from build123d import *

# Parameters (mm, degrees)
SKETCH_W      = 98.2
SKETCH_H      = 92.2
SKETCH_R      = 5
SKETCH_R_2    = 3.2
SKETCH_R_3    = 1.4
SKETCH_R_4    = 2.2
SKETCH_W_2    = 79
SKETCH_H_2    = 52
PAD_DEPTH     = 1.8
SKETCH001_W   = 98.2
SKETCH001_H   = 92.2
SKETCH001_W_2 = 95
SKETCH001_H_2 = 89
PAD001_DEPTH  = 15.7
SKETCH002_R   = 4
SKETCH002_R_2 = 1.55
PAD002_DEPTH  = 6.2
FILLET_R      = 1.79
SKETCH003_W   = 27
SKETCH003_H   = 4
POCKET_DEPTH  = 1.6


with BuildPart() as part:
    # Sketch → Pad (new body)
    with BuildSketch(Plane.XY):
        Rectangle(SKETCH_W, SKETCH_H)
        with Locations((-37, -35)):
            Circle(SKETCH_R, mode=Mode.SUBTRACT)
        with Locations((-4, -35)):
            Circle(SKETCH_R_2, mode=Mode.SUBTRACT)
        with Locations((-23.1, -35)):
            Circle(SKETCH_R_3, mode=Mode.SUBTRACT)
        with Locations((-18.5, -30.4)):
            Circle(SKETCH_R_3, mode=Mode.SUBTRACT)
        with Locations((-13.9, -35)):
            Circle(SKETCH_R_3, mode=Mode.SUBTRACT)
        with Locations((-18.5, -39.6)):
            Circle(SKETCH_R_3, mode=Mode.SUBTRACT)
        with Locations((-18.5, -35)):
            Circle(SKETCH_R_4, mode=Mode.SUBTRACT)
        with Locations((-21.752691, -31.747309)):
            Circle(SKETCH_R_3, mode=Mode.SUBTRACT)
        with Locations((-15.247309, -31.747309)):
            Circle(SKETCH_R_3, mode=Mode.SUBTRACT)
        with Locations((-15.247309, -38.252691)):
            Circle(SKETCH_R_3, mode=Mode.SUBTRACT)
        with Locations((-21.752691, -38.252691)):
            Circle(SKETCH_R_3, mode=Mode.SUBTRACT)
        with Locations((38.5, -31.5)):
            Circle(SKETCH_R_2, mode=Mode.SUBTRACT)
        with Locations((0, 9)):
            Rectangle(SKETCH_W_2, SKETCH_H_2, mode=Mode.SUBTRACT)
    extrude(amount=PAD_DEPTH)

    # Sketch001 → Pad001 (new body)
    with BuildSketch(Plane.XY.offset(1.8)):
        Rectangle(SKETCH001_W, SKETCH001_H)
        Rectangle(SKETCH001_W_2, SKETCH001_H_2, mode=Mode.SUBTRACT)
    extrude(amount=PAD001_DEPTH)

    # Sketch002 → Pad002 (new body)
    with BuildSketch(Plane.XY.offset(1.8)):
        with Locations((-44, 41.5)):
            Circle(SKETCH002_R)
        with Locations((-44, 41.5)):
            Circle(SKETCH002_R_2, mode=Mode.SUBTRACT)
        with Locations((44, 41.5)):
            Circle(SKETCH002_R)
        with Locations((44, 41.5)):
            Circle(SKETCH002_R_2, mode=Mode.SUBTRACT)
        with Locations((44, -24)):
            Circle(SKETCH002_R)
        with Locations((44, -24)):
            Circle(SKETCH002_R_2, mode=Mode.SUBTRACT)
        with Locations((-44, -24)):
            Circle(SKETCH002_R)
        with Locations((-44, -24)):
            Circle(SKETCH002_R_2, mode=Mode.SUBTRACT)
    extrude(amount=PAD002_DEPTH)

    # Fillet
    fillet_edges = [part.edges().sort_by_distance(p)[0] for p in [
        (-49.1, 46.1, 0.9),
        (-49.1, 46.1, 9.65),
        (-49.1, -46.1, 0.9),
        (-49.1, -46.1, 9.65),
        (49.1, 46.1, 0.9),
        (49.1, 46.1, 9.65),
        (49.1, -46.1, 0.9),
        (49.1, -46.1, 9.65),
        (0, -46.1, 0),
        (49.1, 0, 0),
        (0, 46.1, 0),
        (-49.1, 0, 0),
    ]]
    fillet(fillet_edges, radius=FILLET_R)

    # Sketch003 → Pocket (cut)
    with BuildSketch(Plane.YZ.offset(49.1)):
        with Locations((8.5, 15.5)):
            Rectangle(SKETCH003_W, SKETCH003_H)
    extrude(amount=-POCKET_DEPTH, mode=Mode.SUBTRACT)


solid = part.part
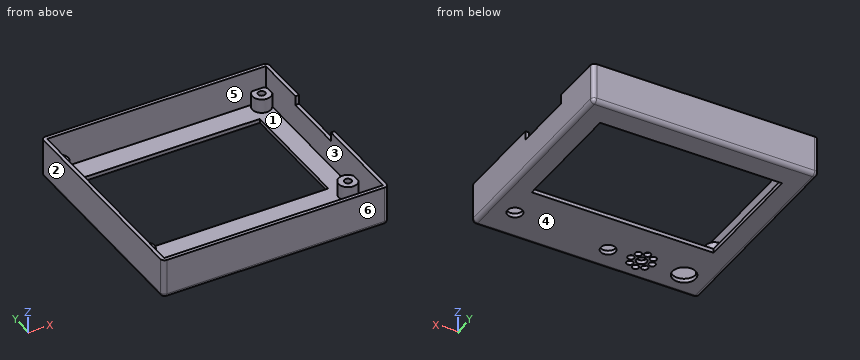
Here's how the part is built. I have some questions about the finished solid (model axes, mm). Face numbers are marked on the shaded views. A direction names the side the tool comes from. Coordinates: 2 decimals unless noted, no trailing zeros. Loops run counter-clockwise (first coordinate to the right, second up) from the corner with the lowest first, then second, coordinate; pieces in that order, holes last.
1. Imagine slicing it at B-B, the plane y = 0. Please give me the cut outline in (x, z), and give its area (3 significant figures).
2. Imagine slicing it at D-D, the plane z = 6.5. Please give me the cut outline in (x, y).
3. If we mould it in two halves opening along Y, with no side actions, what happens to the marked faces 3, 4, 5 and 6? For each: pulls with the +Y half, pulls with the -Y half, needs draft (parallel to the pull), parting line crosses it, or undercut.
4. For P1, Ø1.5, axis at x = -9, y = 32.5, coming from the +Z side; P2, Ø1.4, axis at x = 4, z = 0.5, coming from the -Y side; P3, Ø3.5, axis at x = -44.5, y = 41, coming from the +Z side; P4, Ø0.5, axis at x = 14.5, z = 1, coming from the +Y side, each with a flat end and sliding along its axis, tell me the tip position at first contact or that it passes through.
5. I need wall thicknesses on L1, parallel to Y at x = 44, z = 4; L2, parallel to X at y = -39.5, z = 3.5; L3, parallel to Y at x = 36.5, z = 13.75. Which ranges of each line are inside material? Lowest first, please.
6. Imagine slicing it at C-C, the plane x = 8. Please give me the cut outline in (y, z).
7. Imagine slicing it at A-A, the plane x = -34. Please give me the cut outline in (y, z).
8. For the marked faces 1 and 2, which set-ups out of +Z, -Z, +X, -X, +Y, -Y let a thin tool reach every point of the face, with its end or its side?
Taken from the geometry:
1. outline: (-49.1, 1.79) arc R1.79 ccw to (-47.31, 0) - (-39.5, 0) - (-39.5, 1.8) - (-47.5, 1.8) - (-47.5, 17.5) - (-49.1, 17.5) - close; (39.5, 0) - (47.31, 0) arc R1.79 ccw to (49.1, 1.79) - (49.1, 13.5) - (47.5, 13.5) - (47.5, 1.8) - (39.5, 1.8) - close
1. area: 77.0 mm2
2. outline: (-49.1, -44.31) arc R1.79 ccw to (-47.31, -46.1) - (47.31, -46.1) arc R1.79 ccw to (49.1, -44.31) - (49.1, 44.31) arc R1.79 ccw to (47.31, 46.1) - (-47.31, 46.1) arc R1.79 ccw to (-49.1, 44.31) - close; hole (-47.5, -44.5) - (47.5, -44.5) - (47.5, -25.94) arc R4 cw (long way) to (47.5, -22.06) - (47.5, 39.56) arc R4 cw (long way) to (41.35, 44.5) - (-41.35, 44.5) arc R4 cw (long way) to (-47.5, 39.56) - (-47.5, -22.06) arc R4 cw (long way) to (-47.5, -25.94) - close; hole (-47.5, 43.44) arc R4 cw to (-46.65, 44.5) - (-47.5, 44.5) - close; hole circle Ø3.1 at (-44, -24); hole circle Ø3.1 at (-44, 41.5); hole circle Ø3.1 at (44, -24); hole circle Ø3.1 at (44, 41.5); hole (46.65, 44.5) arc R4 cw to (47.5, 43.44) - (47.5, 44.5) - close
3. face 3: undercut
3. face 4: needs draft
3. face 5: undercut
3. face 6: pulls with the -Y half
4. P1: passes through
4. P2: stops at y = -46
4. P3: stops at z = 8
4. P4: stops at y = 46.02
5. L1: y = -46.1 to -44.5, -28 to -25.55, -22.45 to -20, 37.5 to 39.95, 43.05 to 46.1
5. L2: x = -49.1 to -47.5, 47.5 to 49.1
5. L3: y = -46.1 to -44.5, 44.5 to 46.1
6. outline: (-46.1, 1.79) arc R1.79 ccw to (-44.31, 0) - (-17, 0) - (-17, 1.8) - (-44.5, 1.8) - (-44.5, 17.5) - (-46.1, 17.5) - close; (35, 0) - (44.31, 0) arc R1.79 ccw to (46.1, 1.79) - (46.1, 17.5) - (44.5, 17.5) - (44.5, 1.8) - (35, 1.8) - close
7. outline: (-46.1, 1.79) arc R1.79 ccw to (-44.31, 0) - (-39, 0) - (-39, 1.8) - (-44.5, 1.8) - (-44.5, 17.5) - (-46.1, 17.5) - close; (-31, 0) - (-17, 0) - (-17, 1.8) - (-31, 1.8) - close; (35, 0) - (44.31, 0) arc R1.79 ccw to (46.1, 1.79) - (46.1, 17.5) - (44.5, 17.5) - (44.5, 1.8) - (35, 1.8) - close
8. face 1: +Z
8. face 2: +Z, -Z, -X, +Y, -Y
